```python
from build123d import *

# Parameters (mm, degrees)
F0_W     = 3.175
F0_H     = 3.175
F1_DEPTH = 3.175


# Not quite as in the source:
# - a feature names something its author has since deleted; it is built from what else it names


with BuildPart() as f1:
    # F0 (on Front) → F1 (new body)
    with BuildSketch(Plane.XZ):
        Polygon((-56.6817452915, 14.4236114298), (-56.6817452915, 11.2486114298), (-53.5067452915, 11.2486114298), (-42.3942452915, 11.2486114298), (-23.3442452915, 11.2486114298), (-4.2942452915, 11.2486114298), (6.8182547085, 11.2486114298), (6.8182547085, 14.4236114298), align=None)
        with Locations((-55.0942452915, 9.6611114298)):
            Rectangle(F0_W, F0_H)
        with Locations((-58.2692452915, 6.4861114298)):
            Rectangle(F0_W, F0_H)
        Polygon((-42.3942452915, 11.2486114298), (-53.5067452915, 11.2486114298), (-53.5067452915, 8.0736114298), (-53.5067452915, 4.8986114298), (-53.5067452915, 1.7236114298), (-53.5067452915, -1.4513885702), (-53.5067452915, -4.6263885702), (-53.5067452915, -7.8013885702), (-53.5067452915, -10.9763885702), (-53.5067452915, -14.1513885702), (-53.5067452915, -17.3263885702), (-53.5067452915, -20.5013885702), (-53.5067452915, -23.6763885702), (-53.5067452915, -26.8513885702), (-53.5067452915, -30.0263885702), (-53.5067452915, -33.2013885702), (-53.5067452915, -36.3763885702), (-53.5067452915, -39.5513885702), (-42.3942452915, -39.5513885702), align=None)
        with Locations((-55.0942452915, 6.4861114298)):
            Rectangle(F0_W, F0_H)
        with Locations((-55.0942452915, 3.3111114298)):
            Rectangle(F0_W, F0_H)
        with Locations((-58.2692452915, 0.1361114298)):
            Rectangle(F0_W, F0_H)
        Polygon((-23.3442452915, -39.5513885702), (-42.3942452915, -39.5513885702), (-53.5067452915, -39.5513885702), (-53.5067452915, -42.7263885702), (6.8182547085, -42.7263885702), (6.8182547085, -39.5513885702), (-4.2942452915, -39.5513885702), align=None)
        Polygon((6.8182547085, 8.0736114298), (6.8182547085, 11.2486114298), (-4.2942452915, 11.2486114298), (-4.2942452915, -39.5513885702), (6.8182547085, -39.5513885702), (6.8182547085, -36.3763885702), (6.8182547085, -33.2013885702), (6.8182547085, -30.0263885702), (6.8182547085, -26.8513885702), (6.8182547085, -23.6763885702), (6.8182547085, -20.5013885702), (6.8182547085, -17.3263885702), (6.8182547085, -14.1513885702), (6.8182547085, -10.9763885702), (6.8182547085, -7.8013885702), (6.8182547085, -4.6263885702), (6.8182547085, -1.4513885702), (6.8182547085, 1.7236114298), (6.8182547085, 4.8986114298), align=None)
        with Locations((-55.0942452915, 0.1361114298)):
            Rectangle(F0_W, F0_H)
        with Locations((-55.0942452915, -41.1388885702)):
            Rectangle(F0_W, F0_H)
        with Locations((-55.0942452915, -37.9638885702)):
            Rectangle(F0_W, F0_H)
        with Locations((8.4057547085, 6.4861114298)):
            Rectangle(F0_W, F0_H)
        with Locations((-55.0942452915, -3.0388885702)):
            Rectangle(F0_W, F0_H)
        with Locations((-58.2692452915, -6.2138885702)):
            Rectangle(F0_W, F0_H)
        with Locations((-58.2692452915, -37.9638885702)):
            Rectangle(F0_W, F0_H)
        with Locations((-55.0942452915, -34.7888885702)):
            Rectangle(F0_W, F0_H)
        with Locations((-55.0942452915, -6.2138885702)):
            Rectangle(F0_W, F0_H)
        with Locations((8.4057547085, -37.9638885702)):
            Rectangle(F0_W, F0_H)
        with Locations((-55.0942452915, -31.6138885702)):
            Rectangle(F0_W, F0_H)
        with Locations((8.4057547085, 0.1361114298)):
            Rectangle(F0_W, F0_H)
        with Locations((-55.0942452915, -9.3888885702)):
            Rectangle(F0_W, F0_H)
        with Locations((-58.2692452915, -12.5638885702)):
            Rectangle(F0_W, F0_H)
        with Locations((-58.2692452915, -31.6138885702)):
            Rectangle(F0_W, F0_H)
        with Locations((-55.0942452915, -28.4388885702)):
            Rectangle(F0_W, F0_H)
        with Locations((-55.0942452915, -12.5638885702)):
            Rectangle(F0_W, F0_H)
        with Locations((8.4057547085, -31.6138885702)):
            Rectangle(F0_W, F0_H)
        with Locations((-55.0942452915, -25.2638885702)):
            Rectangle(F0_W, F0_H)
        with Locations((8.4057547085, -6.2138885702)):
            Rectangle(F0_W, F0_H)
        with Locations((-55.0942452915, -15.7388885702)):
            Rectangle(F0_W, F0_H)
        with Locations((-58.2692452915, -18.9138885702)):
            Rectangle(F0_W, F0_H)
        with Locations((-58.2692452915, -25.2638885702)):
            Rectangle(F0_W, F0_H)
        with Locations((-55.0942452915, -22.0888885702)):
            Rectangle(F0_W, F0_H)
        with Locations((-55.0942452915, -18.9138885702)):
            Rectangle(F0_W, F0_H)
        with Locations((8.4057547085, -25.2638885702)):
            Rectangle(F0_W, F0_H)
        with Locations((8.4057547085, -12.5638885702)):
            Rectangle(F0_W, F0_H)
        with Locations((8.4057547085, -18.9138885702)):
            Rectangle(F0_W, F0_H)
    extrude(amount=F1_DEPTH)


solid = f1.part
```
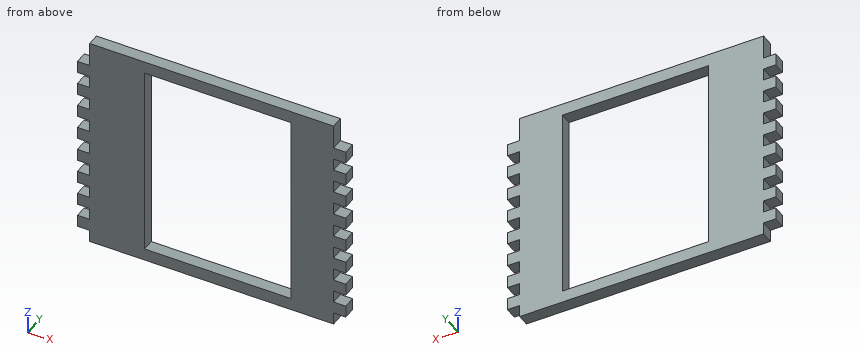
Build history of the part. All positions in model axes, mm. Round coordinates to 2 decimals unless told otherwise and drop trailing zeros. Write each loop counter-clockwise with the first axis right and the second up, starting at its lowest first coordinate (ties: lowest second). Pieces come first, ordered by that corner, then holes. Notation, with made-up numbers: (10, 39.5) -> (66, 39.5) arc R21 ccw to (66, 52.5) -> close; hole circle Ø2 at (-31, 51). An arc over 180 degrees is marked (long way). Put each result on its own line as item: value.
Item 1: Slice it at B-B, the plane z = -28. Give the cut face in (x, y) (3 decimals).
Here are the results:
outline: (-56.682, -3.175) -> (-42.394, -3.175) -> (-42.394, 0) -> (-56.682, 0) -> close; (-4.294, -3.175) -> (6.818, -3.175) -> (6.818, 0) -> (-4.294, 0) -> close
Item 2: Flat gauge pins, fed straight in: P1, Ø1, axis at y = -1.5, z = -3, coming from the -X side; P2, Ø1, axis at y = -1.5, z = -2.5, coming from the +X side; P3, Ø1.6, axis at x = -58, y = -1.5, coming from the -Z side. Where does each tip first touch, or does it go through?
Here are the results:
P1: stops at x = -56.68
P2: stops at x = 6.82
P3: stops at z = -39.55
Item 3: Wall check: probe 1 along Z at (x, y) = (-34.5, -0.65); probe 2 along X at (y, z) = (-0.1, -27); probe 3 along X at (y, z) = (-0.9, -39). Give the ranges that are in metal, low to high. Write a range as from..to.
Here are the results:
probe 1: z = -42.73..-39.55, 11.25..14.42
probe 2: x = -56.68..-42.39, -4.29..6.82
probe 3: x = -59.86..-42.39, -4.29..9.99
Item 4: Slice it at A-A, the plane x = -9.5. Give the cut face in (y, z) (3 decimals).
Here are the results:
outline: (-3.175, -42.726) -> (0, -42.726) -> (0, -39.551) -> (-3.175, -39.551) -> close; (-3.175, 11.249) -> (0, 11.249) -> (0, 14.424) -> (-3.175, 14.424) -> close
